Geometry: final body of the model. Coordinates: model frame, mm. A direction names the side the tool comes from. Give positions to 0.01 mm unless a question says otherwise; leave off trailing zeros. Write each loop counter-clockwise with the first axis right and the second up, starting at its lowest first coordinate (ties: lowest second). Pieces come first, ordered by that corner, then holes.
from build123d import *

# Parameters (mm, degrees)
SKETCH_1_W           = 13.199674752
SKETCH_1_H           = 69.2763861
EXTRUDE_1_DEPTH      = 2
EXTRUDE_2_DEPTH      = 3
EXTRUDE_2_DEPTH_BACK = 5
SKETCH_2_R           = 2.000590496


with BuildPart() as part:
    # 草图1 → 凸台-拉伸1 (new body)
    with BuildSketch(Plane.XY):
        Rectangle(SKETCH_1_W, SKETCH_1_H)
    extrude(amount=EXTRUDE_1_DEPTH)

    # 草图2 → 凸台-拉伸2 (add, two sides: drawn at the far end of the back side and taken through both)
    with BuildSketch(Plane.XY.offset(2).offset(-EXTRUDE_2_DEPTH_BACK)):
        with Locations((0, -26.790353818)):
            Circle(SKETCH_2_R)
    extrude(amount=EXTRUDE_2_DEPTH + EXTRUDE_2_DEPTH_BACK)


solid = part.part
Q1. Section D-D on x = -4. Output: boundary loops of the cut face in (y, z).
Filled sheet:
outline: (-34.64, 0) - (34.64, 0) - (34.64, 2) - (-34.64, 2) - close
Q2. Ray query, line 1 along Z through (x, y) = (-2.75, -24.5); line 2 along X through (y, z) = (-26, -2). Return the intervals inside material, ascending.
Filled sheet:
line 1: z = 0 to 2
line 2: x = -1.84 to 1.84
Q3. Access query for faces 1 (the cylindrical face through (0.923, -28.565, -1.521)), 2 (the flat face through (6.6, 0, 1)), 3 (the cylindrical face through (0.923, -28.565, 3.479)). Directions: +Z, -Z, +X, -X, +Y, -Y. A direction counts if a zero-diameter tool reaches every point of the face in a straight line with its end or side. Return the directions, or none.
Filled sheet:
face 1: -Z
face 2: +Z, -Z, +X, +Y, -Y
face 3: +Z
Q4. Section C-C on z = 3.75. Output: boundary loops of the cut face in (x, y).
Filled sheet:
outline: circle Ø4 at (0, -26.79)
Q5. Section A-A on x = 0. Output: boundary loops of the cut face in (y, z).
Filled sheet:
outline: (-34.64, 0) - (-28.79, 0) - (-28.79, -3) - (-24.79, -3) - (-24.79, 0) - (34.64, 0) - (34.64, 2) - (-24.79, 2) - (-24.79, 5) - (-28.79, 5) - (-28.79, 2) - (-34.64, 2) - close
Q6. Pin query (flat end, axial travel): P1, Ø1, axis at x = -3, z = 3.5, coming from the +Y side; P2, Ø1, axis at x = 2.5, y = 11, coming from the -Z side. Return the tip coordinate at first contact, or that it passes through.
Filled sheet:
P1: passes through
P2: stops at z = 0
Q7. Section B-B on y = 30. Output: boundary loops of the cut face in (x, z).
Filled sheet:
outline: (-6.6, 0) - (6.6, 0) - (6.6, 2) - (-6.6, 2) - close
